Verification items for the finished model (mm, model axes). A direction names the side the tool comes from. Give positions to 0.01 mm unless a question says otherwise; leave off trailing zeros. Write each loop counter-clockwise with the first axis right and the second up, starting at its lowest first coordinate (ties: lowest second). Pieces come first, ordered by that corner, then holes. Notation, with made-up numbers: (82.5, 15) - (97.5, 15) arc R28 cw to (97.5, 34) - close; hole circle Ø8 at (5.5, 76.25). An arc over 180 degrees is marked (long way). Put each result on its own line as item: value.
from build123d import *

# Parameters (mm, degrees)
SKETCH_1_W          = 35
SKETCH_1_H          = 15
EXTRUDE_1_DEPTH     = 6
SKETCH_2_R          = 1.5
CUT_EXTRUDE_1_DEPTH = 16
SKETCH_3_R          = 4.1
CUT_EXTRUDE_2_DEPTH = 7
CUT_EXTRUDE_3_DEPTH = 7


with BuildPart() as part:
    # 草图1 → 凸台-拉伸1 (new body)
    with BuildSketch(Plane(origin=(0, 0, 0), x_dir=(0, 0, -1), z_dir=(1, 0, 0))):
        Rectangle(SKETCH_1_W, SKETCH_1_H)
    extrude(amount=EXTRUDE_1_DEPTH)

    # 草图2 → 切除-拉伸1 (cut, through all)
    with BuildSketch(Plane(origin=(0, 7.5, 0), x_dir=(1, 0, 0), z_dir=(0, 1, 0))):
        with Locations((3, -13.5)):
            Circle(SKETCH_2_R)
        with Locations((3, 1.5)):
            Circle(SKETCH_2_R)
    extrude(amount=-CUT_EXTRUDE_1_DEPTH, mode=Mode.SUBTRACT)

    # 草图3 → 切除-拉伸2 (cut, through all)
    with BuildSketch(Plane(origin=(6, 0, 0), x_dir=(0, 0, -1), z_dir=(1, 0, 0))):
        with Locations((9, -1)):
            Circle(SKETCH_3_R)
    extrude(amount=-CUT_EXTRUDE_2_DEPTH, mode=Mode.SUBTRACT)

    # 草图4 → 切除-拉伸3 (cut, through all)
    with BuildSketch(Plane(origin=(6, 0, 0), x_dir=(0, 0, -1), z_dir=(1, 0, 0))):
        with BuildLine():
            Line((9, 5.1), (9, 7.5))
            Line((9, 7.5), (17.5, 7.5))
            Line((17.5, 7.5), (17.5, -7.5))
            Line((17.5, -7.5), (-17.5, -7.5))
            Line((-17.5, -7.5), (9.091905641, -7.099307613))
            ThreePointArc((9.091905641, -7.099307613), (15.099826901, -0.954045876), (9, 5.1))
        make_face()
    extrude(amount=-CUT_EXTRUDE_3_DEPTH, mode=Mode.SUBTRACT)


solid = part.part
Q1. Section check D-D, the plane x = 0.55. Record the cut outline in (y, z).
Answers follow:
outline: (-7.5, 17.5) - (-7.1, -9.09) arc R6.1 ccw to (5.1, -9) - (7.5, -9) - (7.5, 17.5) - close; hole circle Ø8.2 at (-1, -9)
Q2. Section check C-C, the plane z = 13.5. Record the cut outline in (x, y).
Answers follow:
outline: (0, -7.44) - (1.5, -7.44) - (1.5, 7.5) - (0, 7.5) - close; (4.5, -7.44) - (6, -7.44) - (6, 7.5) - (4.5, 7.5) - close
Q3. Set-up check for faces 4 (the face through (3.806, 0.233, -2.765)), 5 (the face through (3, 6, -9)): record each of +Z, -Z, +X, -X, +Y, -Y from which the full face is reachable in a straight line by a thin tool's end or side.
Answers follow:
face 4: +Y, -Y
face 5: -Z, +X, -X, +Y
Q4. Section check B-B, the plane x = 1.95. Record the cut outline in (y, z), plus the area to 3 significant figures.
Answers follow:
outline: (-7.5, 17.5) - (-7.46, 14.57) - (7.5, 14.57) - (7.5, 17.5) - close; (-7.42, 12.43) - (-7.23, -0.43) - (7.5, -0.43) - (7.5, 12.43) - close; (-7.2, -2.57) - (-7.1, -9.09) arc R6.1 ccw to (5.1, -9) - (7.5, -9) - (7.5, -2.57) - close; hole circle Ø8.2 at (-1, -9)
area: 334 mm2
Q5. Release check for a two-part mould opening along Y. For faces 1 (the face through (3, -1.1, -15.1)), 2 (the face through (3.042, -0.82, -4.904)), 3 (the face through (4.386, 0.121, 14.075)) record: released by +Y, released by -Y, zero draft, split by the parting line, or undercut.
Answers follow:
face 1: split by the parting line
face 2: undercut
face 3: zero draft
Q6. Scan lines: line 1 along X through (y, z) = (-0.25, -1.5); line 2 along Z through (x, y) = (3.1, -4.5); line 3 along Z through (x, y) = (3, 0.75). Record each from-to range of solid material in increasing order.
Answers follow:
line 1: x = 0 to 1.5, 4.5 to 6
line 2: z = -14 to -11.14, -6.86 to -3, 0 to 12, 15 to 17.5
line 3: z = -14.84 to -12.71, -5.29 to -3, 0 to 12, 15 to 17.5
Q7. Section check A-A, the plane y = -1. Record the cut outline in (x, z), plus the area to 3 significant figures.
Answers follow:
outline: (0, -15.1) - (6, -15.1) - (6, -13.1) - (0, -13.1) - close; (0, -4.9) - (6, -4.9) - (6, 17.5) - (0, 17.5) - close; hole circle Ø3 at (3, -1.5); hole circle Ø3 at (3, 13.5)
area: 132 mm2
Q8. Go/stop test with flat-tipped pins: pin 1 Ø1.8 at (x, z) = (3, 13.5) entering from -Y; pin 2 Ø2.5 at (x, y) = (2, 7) entering from -Z; pin 3 Ø2 at (x, y) = (3.5, -1.5) entering from -Z. Record where each tip stops, or that it passes through.
Answers follow:
pin 1: passes through
pin 2: stops at z = -9
pin 3: stops at z = -15.1
